Check sheet for the modelled part. Datum: model origin and axes. Units: mm. A direction names the side the tool comes from. Give positions to 0.01 mm unless a question says otherwise; leave off trailing zeros. Order: outer loops, then holes, each group sorted by start corner. A loop starts at its lowest first (then second) coordinate and runs counter-clockwise, first axis right, second up. Notation, with made-up numbers: M -23.75,-26 L 23.25,-26 A10 cw 23.25,-20 Z; hole C 15.5,24.25 d9. An arc over 180 degrees is marked long. Return JSON: item names as keys, results as strings. Group by question number.
from build123d import *

# Parameters (mm, degrees)
F0_W      = 2240
F0_H      = 1320
F1_DEPTH  = 1020
F3_DEPTH  = 2240.001
F5_DEPTH  = 2240.001
F6_W      = 1007.5
F6_H      = 1045
F7_DEPTH  = 75
F8_W      = 1007.5
F8_H      = 1245
F9_DEPTH  = 75
F10_W     = 2090
F10_H     = 889.4229168149
F11_DEPTH = 75


with BuildPart() as f1:
    # F0 (on Front) → F1 (new body)
    with BuildSketch(Plane.XZ):
        with Locations((1120, 660)):
            Rectangle(F0_W, F0_H)
    extrude(amount=-F1_DEPTH)

    # F2 (on face) → F3 (cut, through all)
    with BuildSketch(Plane(origin=(0, 0, 0), x_dir=(0, -1, 0), z_dir=(-1, 0, 0))):
        Polygon((-1020, 1120), (0, 1320), (-1020, 1320), align=None)
    extrude(amount=-F3_DEPTH, mode=Mode.SUBTRACT)

    # F4 (on face) → F5 (cut, through all)
    with BuildSketch(Plane(origin=(0, 0, 0), x_dir=(0, -1, 0), z_dir=(-1, 0, 0))):
        Polygon((-945, 0), (-75, 0), (-75, 1228.8659619989), (-945, 1058.2777267048), align=None)
    extrude(amount=-F5_DEPTH, mode=Mode.SUBTRACT)

    # F6 (on face) → F7 (cut, through all)
    with BuildSketch(Plane(origin=(0, 1020, 0), x_dir=(-1, 0, 0), z_dir=(0, 1, 0))):
        with Locations((-1661.25, 522.5)):
            Rectangle(F6_W, F6_H)
        with Locations((-578.75, 522.5)):
            Rectangle(F6_W, F6_H)
    extrude(amount=-F7_DEPTH, mode=Mode.SUBTRACT)

    # F8 (on face) → F9 (cut)
    with BuildSketch(Plane.XZ):
        with Locations((578.75, 622.5)):
            Rectangle(F8_W, F8_H)
        with Locations((1661.25, 622.5)):
            Rectangle(F8_W, F8_H)
    extrude(amount=-F9_DEPTH, mode=Mode.SUBTRACT)

    # F10 (on face) → F11 (cut)
    with BuildSketch(Plane(origin=(0, 249.2410218438, 1271.1292114032), x_dir=(1, 0, 0), z_dir=(0, 0.1924144607, 0.9813137497))):
        with Locations((1120, 265.7243702557)):
            Rectangle(F10_W, F10_H)
    extrude(amount=-F11_DEPTH, mode=Mode.SUBTRACT)


solid = f1.part
1) Release check for a two-part mould opening along X. For faces 1 (the face through (572, 30, 1245)), 2 (the face through (0, 508, 1146)), 3 (the face through (1115, 945, 532)), 4 (the face through (1105.37, 68.087, 1277.462)) record: released by +X, released by -X, zero draft, split by the parting line, or undercut.
2) Depth check by flat-ended pin: P1, Ø18.5, axis at x = 1657.5, y = 45.5, coming from the -Z side; P2, Ø8, axis at x = 838, z = 1074.5, coming from the -Y side. Enter the tip coordinate at first touch or a pass-through.
3) Sectioned sample at C-C on y = 175. Record the boundary of the cut face in (x, z).
4) Tool access check on faces 5 (the face through (36.25, 507.97, 1143.97)), 6 (the face through (1031.81, 965.713, 1130.644)), 7 (the face through (1119, 75, 606)), 8 (the face through (1654, 30, 1245)). Record the directions out of +Z, -Z, +X, -X, +Y, -Y that give a thin tool (end or side, any length) a straight path to the whole face; none if there is none.
5) Material ranges on line 1 along X through (y, z) = (68.5, 1093.5), recorded low to high.
6) Sectioned sample at A-A on x = 1454. Record the boundary of the cut face in (y, z), then the cut area to 4 significant figures.
7) Sectioned sample at B-B on z = 324.5. Record the boundary of the cut face in (x, y).
Reply:
{
 "1": {"face 1": "undercut", "face 2": "released by -X", "face 3": "zero draft", "face 4": "undercut"},
 "2": {"P1": "z = 1245", "P2": "y = 933.87"},
 "3": {"outline": "M 0,1209.26 L 75,1209.26 L 75,1285.69 L 0,1285.69 Z; M 2165,1209.26 L 2240,1209.26 L 2240,1285.69 L 2165,1285.69 Z"},
 "4": {"face 5": "-Z, +X, -X", "face 6": "+Z, +X, -X, +Y", "face 7": "+Z, -Z, +X, -X", "face 8": "-Z, +Y, -Y"},
 "5": {"line 1": "0 to 75, 1082.5 to 1157.5, 2165 to 2240"},
 "6": {"outline": "M 0,1245 L 61.72,1245 L 73.6,1305.57 L 0,1320 Z; M 931.97,1060.83 L 945,1058.28 L 945,1045 L 1020,1045 L 1020,1120 L 946.4,1134.43 Z", "area": "11,250 mm^2"},
 "7": {"outline": "M 0,0 L 75,0 L 75,75 L 0,75 Z; M 0,945 L 75,945 L 75,1020 L 0,1020 Z; M 1082.5,0 L 1157.5,0 L 1157.5,75 L 1082.5,75 Z; M 1082.5,945 L 1157.5,945 L 1157.5,1020 L 1082.5,1020 Z; M 2165,0 L 2240,0 L 2240,75 L 2165,75 Z; M 2165,945 L 2240,945 L 2240,1020 L 2165,1020 Z"}
}
